Source: CAD feature listing. Evaluate the final solid. Frame: model axes, mm. A direction names the side the tool comes from. Give positions to 0.01 mm unless a question says otherwise; leave off trailing zeros. Write each loop counter-clockwise with the first axis right and the second up, starting at its lowest first coordinate (ties: lowest second). Pieces come first, ordered by that corner, then holes. Notation, with made-up numbers: (-11.5, 24.5) -> (33.5, 24.5) arc R19 ccw to (33.5, 43.5) -> close; hole circle Ø9 at (14, -30.5). An arc over 180 degrees is marked (long way). Write item = value, one per line.
Autodesk Inventor part; units mm, degrees
ref_plane "Work Plane1" through (12.4714, -20.7772, 29.8196) normal (0, 1, 0) x (0, 0, 1)
ref_plane "Work Plane2" through (12.4714, -20.7772, 29.8196) normal (0, 1, 0) x (0, 0, 1)
ref_plane "YZ Plane" through (0, 0, 0) normal (1, 0, 0) x (0, 1, 0)
sketch "Sketch1" plane through (0, 0, 0) normal (0, 0, 1) x (1, 0, 0)
  line L0 (38.1, -31.75) -> (-38.1, -31.75)
  line L1 (-38.1, -31.75) -> (-38.1, 31.75)
  line L2 (-38.1, 31.75) -> (38.1, 31.75)
  line L3 (38.1, 31.75) -> (38.1, -31.75)
  line L4 (38.1, -31.75) -> (-38.1, 31.75) construction
  line L5 (-38.1, -31.75) -> (38.1, 31.75) construction
  point P0 (0, 0)
  dimension "d0" = 76.2
  dimension "d1" = 63.5
extrude "Extrusion1" add sketch "Sketch1" along normal blind 6.35
sketch "Sketch2" plane through (0, 0, 6.35) normal (0, 0, 1) x (1, 0, 0)
  line L0 (-38.1, -31.75) -> (38.1, -31.75)
  line L1 (38.1, -31.75) -> (38.1, 31.75)
  line L2 (-38.1, -31.75) -> (38.1, -31.75)
  line L3 (38.1, -31.75) -> (38.1, -25.4)
  line L4 (38.1, -25.4) -> (-38.1, -25.4)
  line L5 (-38.1, -25.4) -> (-38.1, -31.75)
  point P0 (0, 0)
  dimension "d4" = 6.35
extrude "Extrusion2" add sketch "Sketch2" along normal blind 57.15
fillet "Fillet1" radius 12.7 4 edges at (38.1, 31.75, 3.175) (-38.1, 31.75, 3.175) (38.1, -28.575, 63.5) (-38.1, -28.575, 63.5)
sketch "Sketch3" plane through (0, 0, 6.35) normal (0, 0, 1) x (1, 0, 0)
  circle A0 centre (0, 0) radius 3.175
  dimension "d8" = 6.35
extrude "Extrusion3" cut sketch "Sketch3" against normal blind 25.4
sketch "Sketch4" plane through (-38.1, -25.4, 6.35) normal (0, 1, 0) x (1, 0, 0)
  line L0 (69.85, -20.2184) -> (69.85, -31.5468)
  line L1 (54.1906, -20.0152) -> (69.6468, -20.0152)
  line L2 (47.1932, -24.362) -> (47.1932, -20.2184)
  line L3 (47.1932, -31.5468) -> (47.1932, -27.4032)
  line L4 (69.6468, -31.75) -> (54.1906, -31.75)
  line L5 (51.7782, -31.75) -> (47.3964, -31.75)
  line L6 (69.85, -31.5468) -> (69.85, -31.75)
  line L7 (69.85, -31.75) -> (69.6468, -31.75)
  line L8 (69.6468, -31.75) -> (47.1932, -31.75)
  line L9 (47.1932, -31.75) -> (47.1932, -20.0152)
  line L10 (47.1932, -20.0152) -> (69.85, -20.0152)
  line L11 (69.85, -20.0152) -> (69.85, -31.5468)
  arc A0 (73.6332, -25.2857) -> (73.6332, -26.4795) centre (72.4408, -25.8826) ccw
  circle A1 centre (72.4408, -25.8826) radius 1.3335
  arc A2 (43.41, -26.4795) -> (43.41, -25.2857) centre (44.6024, -25.8826) ccw
  circle A3 centre (44.6024, -25.8826) radius 1.3335
  point P0 (38.1, 6.35)
  point P1 (47.1932, -27.4032)
  point P2 (73.6332, -25.2857)
  point P3 (43.41, -25.2857)
  dimension "d11" = 22.6568
extrude "Extrusion4" cut sketch "Sketch4" against normal blind 25.4
sketch "Sketch5" plane through (-38.1, -25.4, 6.35) normal (0, 1, 0) x (1, 0, 0)
  circle A0 centre (23.6728, -25.8826) radius 2.413
  circle A1 centre (52.9844, -25.8826) radius 2.413
  line L0 (76.2, -25.8826) -> (0, -25.8826)
  circle A2 centre (23.6728, -25.8826) radius 0.8255
  circle A3 centre (52.9844, -25.8826) radius 0.8255
  point P0 (38.1, 6.35)
  dimension "d14" = 4.826
ref_plane "Work Plane1" through (12.4714, -20.7772, 29.8196) normal (0, 1, 0) x (0, 0, 1)
ref_plane "Work Plane2" through (12.4714, -20.7772, 29.8196) normal (0, 1, 0) x (0, 0, 1)
extrude "Extrusion5" add sketch "Sketch5" along normal up to surface (4.6228 mm away) contours L0 A2 A0 | A0 L0 A2
properties part number "Base"
1) Cut plane C-C (x = 23). Return the cut outline in (y, z), then the cut area to 3 significant figures.
Computed:
outline = (-31.75, 0) -> (31.75, 0) -> (31.75, 6.35) -> (-25.4, 6.35) -> (-25.4, 26.37) -> (-31.75, 26.37) -> close; (-31.75, 38.1) -> (-25.4, 38.1) -> (-25.4, 63.5) -> (-31.75, 63.5) -> close
area = 692 mm²
2) Cut plane D-D (x = -9). Return the cut outline in (y, z), then the cut area to 3 significant figures.
Computed:
outline = (-31.75, 0) -> (31.75, 0) -> (31.75, 6.35) -> (-25.4, 6.35) -> (-25.4, 63.5) -> (-31.75, 63.5) -> close
area = 766 mm²
3) Access query for faces 4 (the flat face through (21, -29, 38.1)), 5 (the cylindrical face through (34.48, 27.93, 3.22)), 6 (the flat face through (-13, -20.777, 32)), 7 (the flat face through (-1, -7, 0)), 8 (the cylindrical face through (-14.741, -23.121, 34.625)). Directions: +Z, -Z, +X, -X, +Y, -Y. A direction counts if a zero-diameter tool reaches every point of the face in a straight line with its end or side. Return the directions, or none.
Computed:
face_4 = +Y, -Y
face_5 = +Z, -Z, +X, +Y
face_6 = +Z, +X, -X, +Y
face_7 = -Z, +X, -X, +Y, -Y
face_8 = +Y
4) Cut plane B-B (y = 0). Return the cut outline in (x, z) (3 decimals).
Computed:
outline = (-38.1, 0) -> (-3.175, 0) -> (-3.175, 6.35) -> (-38.1, 6.35) -> close; (3.175, 0) -> (38.1, 0) -> (38.1, 6.35) -> (3.175, 6.35) -> close
5) Material intervals for L1, parallel to Y at x = 0, z = 4 (3 decimals); L2, parallel to Z at x = 20, y = -22.5; L3, parallel to Y at x = 12.5, z = 44.5, sorted ascending.
Computed:
L1 = -31.75 to -3.175, 3.175 to 31.75
L2 = 0 to 6.35
L3 = -31.75 to -25.4
6) Draft query along Y for faces 1 (the cylindrical face through (34.28, -28.53, 59.88)), 2 (the flat face through (1, -31.75, 31)), 3 (the cylindrical face through (-0.69, -3.1, 3.22)). Return one class per face: pulls with the +Y half, pulls with the -Y half, needs draft (parallel to the pull), parting line crosses it, or undercut.
Computed:
face_1 = needs draft
face_2 = pulls with the -Y half
face_3 = undercut
7) Contact query for flat-ended pins moving along their axis: pin 1 (8 mm diameter, centred on x = -29, y = -9, fed in from +Z); pin 2 (17 mm diameter, centred on x = -10.5, z = 34.5, fed in from +Y); pin 3 (10 mm diameter, centred on x = -27.5, z = 21, fed in from +Y). Output: stop coordinate, or through.
Computed:
pin_1 = 6.35
pin_2 = -20.78
pin_3 = -25.4
8) Cut plane A-A (x = 0). Return the cut outline in (y, z) (3 decimals).
Computed:
outline = (-31.75, 0) -> (-3.175, 0) -> (-3.175, 6.35) -> (-25.4, 6.35) -> (-25.4, 63.5) -> (-31.75, 63.5) -> close; (3.175, 0) -> (31.75, 0) -> (31.75, 6.35) -> (3.175, 6.35) -> close
